For this review, use the dimensioned drawing (mm, ordinates from the lowest corner) and the shaded views. A direction names the side the tool comes from. Round coordinates to 2 decimals unless told otherwise and drop trailing zeros. Loops run counter-clockwise (first coordinate to the right, second up) from the corner with the lowest first, then second, coordinate; pieces in that order, holes last. Notation, with made-up numbers: (47.25, 56.25) - (93.25, 56.25) arc R25 ccw to (93.25, 77.25) - close; hole circle Ø4 at (13.25, 59.25). An arc over 180 degrees is marked (long way). Answer as CSV lines item,"result". Start each with the question number.
(1) For P1, Ø4.5, axis at x = 1, y = 5, coming from the +Z side; P2, Ø3, axis at y = 6, z = 19, coming from the +X side; P3, Ø2, axis at x = 3, y = 4.5, coming from the -Z side; P4, Ø3, axis at y = 7, z = 15.5, coming from the -X side, all flat-tipped, find the tip position at first contact; note any pin that passes through.
(2) Consider section A-A (x = 27.45). Give the boundary of the cut face in (y, z), and give its area (3 significant figures).
(3) Consider section C-C (x = 15.45). Give the boundary of the cut face in (y, z), and give its area (3 significant figures).
(4) Consider section B-B (y = 3.75). Give the boundary of the cut face in (x, z), and give its area (3 significant figures).
(5) Wall thickness on L1, parallel to Y at x = 1.95, z = 16.3; L2, parallel to X at y = 8.5, z = 7; L3, parallel to Z at x = 2, y = 11.25: over which ranges is each line inside the solid? List them lowest first.
(6) For the marked faces 1, 2, 3 and 4, list the 3-axis set-ups (+Z, -Z, +X, -X, +Y, -Y) from which the entire face can be reached by the end or side of a thin tool; tool diameter is ignored.
(7) Consider section D-D (z = 7.25). Give the boundary of the cut face in (x, y), and give its area (3 significant figures).
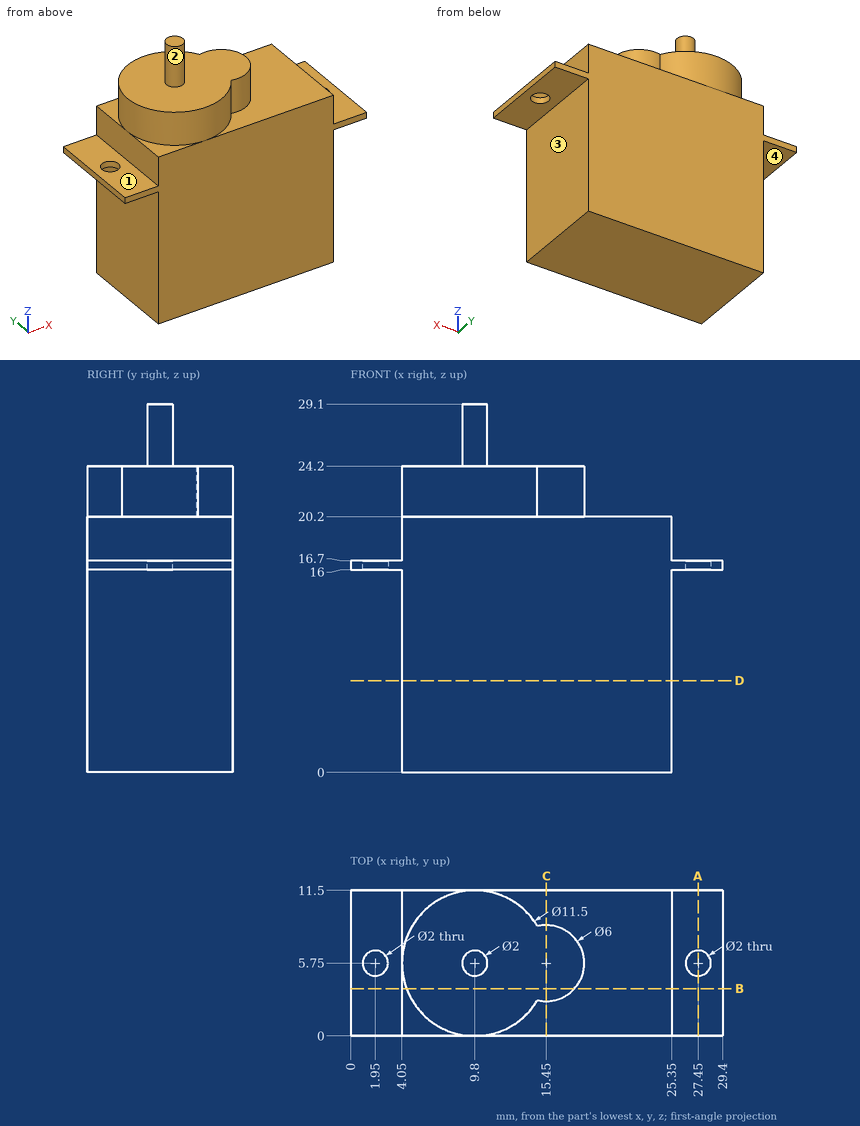
Determined:
1,P1,"stops at z = 16.7"
1,P2,"stops at x = 25.35"
1,P3,"stops at z = 16"
1,P4,"stops at x = 0"
2,outline,"(0, 16) - (4.75, 16) - (4.75, 16.7) - (0, 16.7) - close; (6.75, 16) - (11.5, 16) - (11.5, 16.7) - (6.75, 16.7) - close"
2,area,"6.65 mm^2"
3,outline,"(0, 0) - (11.5, 0) - (11.5, 20.2) - (8.75, 20.2) - (8.75, 24.2) - (2.75, 24.2) - (2.75, 20.2) - (0, 20.2) - close"
3,area,"256 mm^2"
4,outline,"(0, 16) - (4.05, 16) - (4.05, 0) - (25.35, 0) - (25.35, 16) - (29.4, 16) - (29.4, 16.7) - (25.35, 16.7) - (25.35, 20.2) - (17.69, 20.2) - (17.69, 24.2) - (4.41, 24.2) - (4.41, 20.2) - (4.05, 20.2) - (4.05, 16.7) - (0, 16.7) - close"
4,area,"489 mm^2"
5,L1,"y = 0 to 4.75, 6.75 to 11.5"
5,L2,"x = 4.05 to 25.35"
5,L3,"z = 16 to 16.7"
6,face 1,"+Z, -X, +Y, -Y"
6,face 2,"+Z"
6,face 3,"-Z, +X, +Y, -Y"
6,face 4,"-Z, -X, +Y, -Y"
7,outline,"(4.05, 0) - (25.35, 0) - (25.35, 11.5) - (4.05, 11.5) - close"
7,area,"245 mm^2"
